Drawing for the job (mm, zero at the part's lowest x, y, z). A direction names the side the tool comes from. Coordinates: 2 decimals unless noted, no trailing zeros. Write each loop counter-clockwise with the first axis right and the second up, starting at its lowest first coordinate (ties: lowest second). Pieces come first, ordered by that corner, then holes. Notation, with made-up numbers: (41, 10) -> (45, 10) arc R11 ccw to (45, 26) -> close; hole circle Ø9 at (-28.5, 74). An arc over 180 degrees is marked (long way). Answer as CSV lines item,"result".
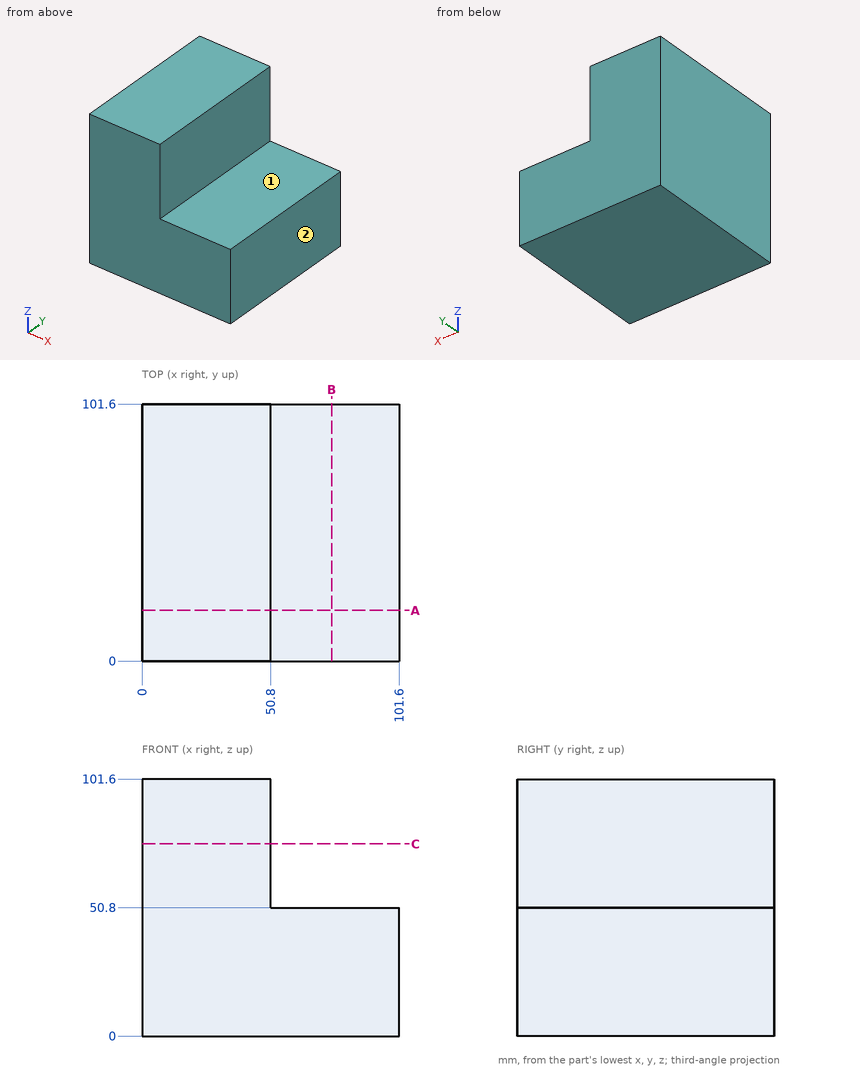
Item 1: 3-axis set-ups, long thin cutter, end or side, ignore diameter. For the marked faces 1 and 2: which of +Z, -Z, +X, -X, +Y, -Y reach the whole face in a straight line?
Answer below:
face 1,"+Z, +X, +Y, -Y"
face 2,"+Z, -Z, +X, +Y, -Y"
Item 2: Flat gauge pins, fed straight in: pin 1 (6 mm diameter, centred on y = 49, z = 77.5, fed in from +X); pin 2 (3 mm diameter, centred on x = 80, z = 53, fed in from -Y). Where does each tip first touch, or does it go through?
Answer below:
pin 1,"stops at x = 50.8"
pin 2,"passes through"
Item 3: Saw through at A-A on y = 20. Give the cut face in (x, z), and give its area (3 significant figures).
Answer below:
outline,"(0, 0) -> (101.6, 0) -> (101.6, 50.8) -> (50.8, 50.8) -> (50.8, 101.6) -> (0, 101.6) -> close"
area,"7,740 mm2"
Item 4: Wall check: line 1 (Z direction, x = 97, y = 55). Give the ranges that are in metal, low to high. Write a range as from..to.
Answer below:
line 1,"z = 0..50.8"
Item 5: Saw through at B-B on x = 75. Give the cut face in (y, z).
Answer below:
outline,"(0, 0) -> (101.6, 0) -> (101.6, 50.8) -> (0, 50.8) -> close"
Item 6: Saw through at C-C on z = 76. Give the cut face in (x, y), and give its area (3 significant figures).
Answer below:
outline,"(0, 0) -> (50.8, 0) -> (50.8, 101.6) -> (0, 101.6) -> close"
area,"5,160 mm2"
